CAD build for the part. Positions are in the model's coordinates, mm. Face numbers are marked on the shaded views. A direction names the side the tool comes from. Round coordinates to 2 decimals unless told otherwise and drop trailing zeros. Write each loop counter-clockwise with the first axis right and the second up, starting at its lowest first coordinate (ties: lowest second). Pieces come first, ordered by that corner, then holes. Notation, with made-up numbers: (-27, -35) - (10, -35) arc R7 cw to (10, -23) - close; hole circle Ø6 at (-32, 86.25). An arc over 180 degrees is marked (long way). Use one line per item in the form item = value. Start each with the question number.
Item 1: Band-saw the part on A-A, the plane z = 0. List the corners of the cut face in (x, y).
Item 2: Band-saw the part on D-D, the plane y = -24.5. List the corners of the cut face in (x, z) (3 decimals).
Item 3: Tool access for the marked faces 4, 5 and 6: list every direction of +Z, -Z, +X, -X, +Y, -Y with a clear straight run to the whole face (end or side of a thin tool).
Item 4: Drill centre lines: L1, parallel to Y at x = 3.25, z = 0; L2, parallel to Y at x = -2.25, z = 0; L3, parallel to X at y = -12, z = -28.5. Where is each one in solid material? Low to high.
Item 5: Pin check, flat tips, straight feed: pin 1 (11 mm diameter, centred on y = 0, z = 0, fed in from -X); pin 2 (4 mm diameter, centred on x = 5, y = -16, fed in from -Z); pin 3 (2 mm diameter, centred on x = 4.5, y = 10, fed in from -Z); pin 4 (3 mm diameter, centred on x = 1.5, y = 13, fed in from -Z). Stop position of each tip, or through.
Item 6: Pull direction Y, two halves, no side cores. Call the marked faces 1, 2 and 3: +Y half, -Y half, draft (parallel to the pull), parting line (faces both ways), or undercut.
Item 7: Band-saw the part on C-C, the plane x = -4.25. List the corners of the cut face in (y, z).
from build123d import *

# Parameters (mm, degrees)
SKETCH1_R                          = 30
CORPO_DA_RODA_DEPTH                = 7.5
SKETCH8_R                          = 35
BOSS_EXTRUDE2_DEPTH                = 2.5
FURO_DO_HUB_MESMO_DI_METRO_1_0_1_D = 12


with BuildPart() as part:
    # Sketch1 → Corpo da Roda (new, symmetric)
    with BuildSketch(Plane(origin=(0, 0, 0), x_dir=(0, 0, -1), z_dir=(1, 0, 0))):
        Circle(SKETCH1_R)
    extrude(amount=CORPO_DA_RODA_DEPTH, both=True)

    # Sketch8 → Boss-Extrude2 (add, symmetric)
    with BuildSketch(Plane(origin=(0, 0, 0), x_dir=(0, 0, -1), z_dir=(1, 0, 0))):
        Circle(SKETCH8_R)
    extrude(amount=BOSS_EXTRUDE2_DEPTH, both=True)

    # Furo do Hub (mesmo diâmetro) - Ø1.0 (1) Diameter Hole1 (through all)
    with Locations(Plane(origin=(7.5, 0, 0), x_dir=(0, 0, -1), z_dir=(1, 0, 0))):
        with Locations((0, 0)):
            Hole(FURO_DO_HUB_MESMO_DI_METRO_1_0_1_D / 2)


solid = part.part
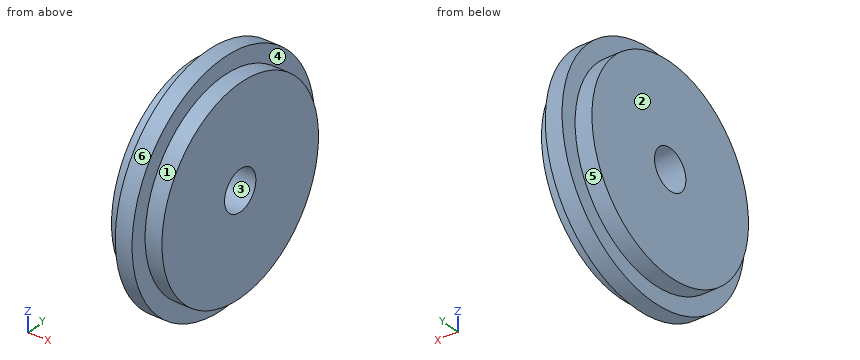
Determined:
q1.outline = (-7.5, -30) - (-2.5, -30) - (-2.5, -35) - (2.5, -35) - (2.5, -30) - (7.5, -30) - (7.5, -6) - (-7.5, -6) - close; (-7.5, 6) - (7.5, 6) - (7.5, 30) - (2.5, 30) - (2.5, 35) - (-2.5, 35) - (-2.5, 30) - (-7.5, 30) - close
q2.outline = (-7.5, -17.313) - (-2.5, -17.313) - (-2.5, -24.995) - (2.5, -24.995) - (2.5, -17.313) - (7.5, -17.313) - (7.5, 17.313) - (2.5, 17.313) - (2.5, 24.995) - (-2.5, 24.995) - (-2.5, 17.313) - (-7.5, 17.313) - close
q3.face_4 = +X
q3.face_5 = -X
q3.face_6 = +X, -X
q4.L1 = -30 to -6, 6 to 30
q4.L2 = -35 to -6, 6 to 35
q4.L3 = -2.5 to 2.5
q5.pin_1 = through
q5.pin_2 = -26.53
q5.pin_3 = -28.62
q5.pin_4 = -33.06
q6.face_1 = parting line
q6.face_2 = draft
q6.face_3 = undercut
q7.outline = circle Ø60 at (0, 0); hole circle Ø12 at (0, 0)
